Part print with two shaded views. Sizes in mm from the minimum x, y, z corner. A direction names the side the tool comes from. Give positions to 0.01 mm unless a question says otherwise; leave off trailing zeros. Write each loop counter-clockwise with the first axis right and the second up, starting at its lowest first coordinate (ties: lowest second). Pieces come first, ordered by that corner, then holes. Notation, with made-up numbers: (46.25, -1) -> (80.25, -1) arc R20 ccw to (80.25, 37) -> close; hole circle Ø10 at (28.5, 2.25). An arc over 180 degrees is marked (long way). Answer as a JSON object with one key per item and string values.
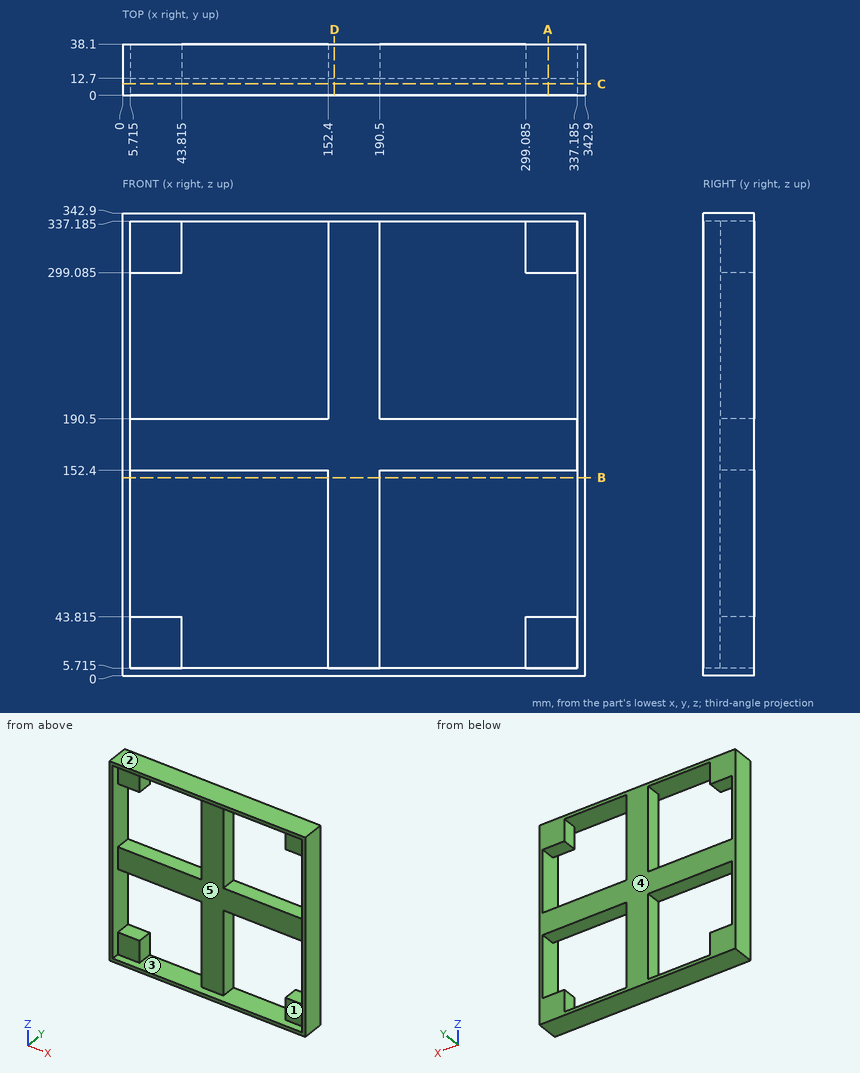
1) Slice it at D-D (x = 157). List the corners of the cut face in (y, z) (3 decimals), then the cut area to 3 significant figures.
Model answer:
{"outline": "(0, 0) -> (38.1, 0) -> (38.1, 342.9) -> (0, 342.9) -> (0, 337.185) -> (12.7, 337.185) -> (12.7, 5.715) -> (0, 5.715) -> close", "area": "8,850 mm2"}
2) Slice it at A-A (x = 315.5). List the corners of the cut face in (y, z) (3 decimals).
Model answer:
{"outline": "(0, 0) -> (38.1, 0) -> (38.1, 43.815) -> (12.7, 43.815) -> (12.7, 5.715) -> (0, 5.715) -> close; (0, 337.185) -> (12.7, 337.185) -> (12.7, 299.085) -> (38.1, 299.085) -> (38.1, 342.9) -> (0, 342.9) -> close; (12.7, 152.4) -> (38.1, 152.4) -> (38.1, 190.5) -> (12.7, 190.5) -> close"}
3) Wall check: probe 1 along Z at (x, y) = (234, 27) (3 decimals); probe 2 along X at (y, z) = (18, 23.5) (3 decimals). Give the ranges that are in metal, low to high.
Model answer:
{"probe 1": "z = 0 to 5.715, 152.4 to 190.5, 337.185 to 342.9", "probe 2": "x = 0 to 43.815, 152.4 to 190.5, 299.085 to 342.9"}
4) Slice it at B-B (z = 147). List the corners of the cut face in (x, y) (3 decimals), then the cut area to 3 significant figures.
Model answer:
{"outline": "(0, 0) -> (5.715, 0) -> (5.715, 38.1) -> (0, 38.1) -> close; (152.4, 12.7) -> (190.5, 12.7) -> (190.5, 38.1) -> (152.4, 38.1) -> close; (337.185, 0) -> (342.9, 0) -> (342.9, 38.1) -> (337.185, 38.1) -> close", "area": "1,400 mm2"}
5) Pin check, flat tip, straight feed: pin 1 (19 mm diameter, centred on x = 311, z = 314, fed in from -Y). Stop position of the tip, or through.
Model answer:
{"pin 1": "stops at y = 12.7"}
6) Slice it at C-C (y = 8.5). List the corners of the cut face in (x, z) (3 decimals), then the cut area to 3 significant figures.
Model answer:
{"outline": "(0, 0) -> (342.9, 0) -> (342.9, 342.9) -> (0, 342.9) -> close; hole (5.715, 5.715) -> (337.185, 5.715) -> (337.185, 337.185) -> (5.715, 337.185) -> close", "area": "7,710 mm2"}
7) 3-axis set-ups, long thin cutter, end or side, ignore diameter. For the marked faces 1 and 2: which of +Z, -Z, +X, -X, +Y, -Y reach the whole face in a straight line?
Model answer:
{"face 1": "-Y", "face 2": "+Z, +X, -X, +Y, -Y"}
8) Mould opens along X. For the marked faces 3, 4 and 5 say: released by +X, released by -X, zero draft, split by the parting line, or undercut.
Model answer:
{"face 3": "undercut", "face 4": "zero draft", "face 5": "undercut"}
